Part model, mm, in its own coordinate system. Face numbers are marked on the shaded views. A direction names the side the tool comes from. Round coordinates to 2 decimals unless told otherwise and drop trailing zeros. Write each loop counter-clockwise with the first axis right and the second up, starting at its lowest first coordinate (ties: lowest second). Pieces come first, ordered by that corner, then holes. Notation, with made-up numbers: (55.5, -20) -> (85.5, -20) arc R21 cw to (85.5, -3) -> close; hole circle Ø5 at (26, 61). An arc over 180 degrees is marked (long way). Return JSON: item names as keys, results as strings. Group by question number.
(1) Mould opens along Y. For the marked faces 1, 2 and 3 say: +Y half, -Y half, draft (parallel to the pull), parting line (faces both ways), or undercut.
(2) Tool access for the marked faces 4, 5, 6 and 7: list every direction of +Z, -Z, +X, -X, +Y, -Y with a clear straight run to the whole face (end or side of a thin tool).
(3) Saw through at C-C (x = 165). List the corners of the cut face in (y, z).
(4) Saw through at B-B (x = 75.5). State how many separate pieces and enclosed holes the cut face has, plus the area to 4 significant figures.
(5) Saw through at A-A (z = 12.5). List the corners of the cut face in (x, y).
(6) Drill centre lines: L1, parallel to Y at x = 13.5, z = 29; L2, parallel to Y at x = 13, z = 6.5; L3, parallel to Y at x = 127, z = 57. Where is each one in solid material? Low to high. Write a range as from..to.
(7) Drop flat-ended pins along their axis: pin 1 Ø6 at (x, z) = (-49, 92) entering from +Y; pin 2 Ø4 at (x, y) = (32, 43.5) entering from +Z; pin 3 Ø2 at (x, z) = (168, 18) entering from +Y; pin 4 Ø12 at (x, y) = (17.5, -7) entering from -Z. Give the stop position or say it passes through.
from build123d import *

# Parameters (mm, degrees)
F3_DEPTH = 100
F4_R     = 8.65938
F4_R_2   = 13.370559
F5_DEPTH = 200


with BuildPart() as f1:
    # F0 (on Front) → F1 (revolve)
    with BuildSketch(Plane.XZ):
        Polygon((0, 112.481035), (0, 0), (58.373801, 0), (58.373801, 42.910885), (103.36262, 57.920542), align=None)
    revolve(axis=Axis((0, 0, 56.240518), (0, 0, -1)))

    # F2 (on face) → F3 (cut)
    with BuildSketch(Plane(origin=(0, 0, 0), x_dir=(1, 0, 0), z_dir=(0, 0, -1))):
        with BuildLine():
            Line((0, 28.951159), (0, -28.951159))
            Line((0, -28.951159), (50.68857, -28.951159))
            ThreePointArc((50.68857, -28.951159), (56.419789, -14.976919), (58.373801, 0))
            ThreePointArc((58.373801, 0), (56.419789, 14.976919), (50.68857, 28.951159))
            Line((50.68857, 28.951159), (0, 28.951159))
        make_face()
        with BuildLine():
            ThreePointArc((58.373801, 0), (56.419789, -14.976919), (50.68857, -28.951159))
            Line((50.68857, -28.951159), (267.143011, -28.951159))
            Line((267.143011, -28.951159), (267.143011, 28.951159))
            Line((267.143011, 28.951159), (50.68857, 28.951159))
            ThreePointArc((50.68857, 28.951159), (56.419789, 14.976919), (58.373801, 0))
        make_face()
    extrude(amount=-F3_DEPTH, mode=Mode.SUBTRACT)

    # F4 (on face) → F5 (join)
    with BuildSketch(Plane.YZ):
        with Locations((-9.289023, 57.48608)):
            Circle(F4_R)
        with Locations((-7.069625, 20.480426)):
            Circle(F4_R_2)
    extrude(amount=F5_DEPTH)


solid = f1.part
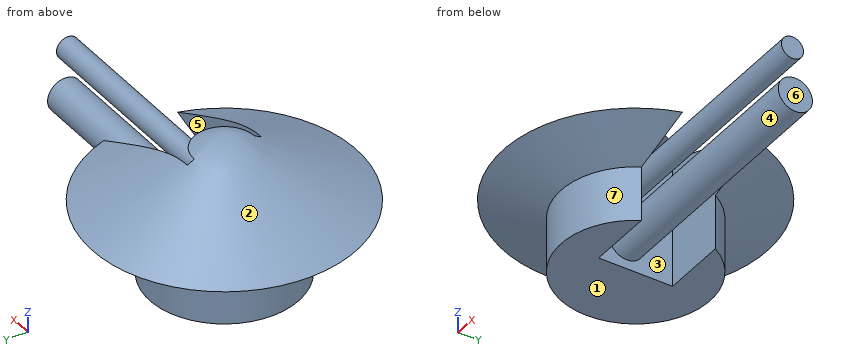
Computed values:
{
 "1": {"face 1": "draft", "face 2": "parting line", "face 3": "undercut"},
 "2": {"face 4": "+X", "face 5": "+Z, -Z, +X", "face 6": "+Z, -Z, +X, +Y, -Y", "face 7": "-Z"},
 "3": {"outline": "circle Ø26.74 at (-7.07, 20.48); circle Ø17.32 at (-9.29, 57.49)"},
 "4": {"separate pieces": "4", "enclosed holes": "0", "area": "1,685 mm2"},
 "5": {"outline": "(0, -28.95) -> (0, -17.8) -> (200, -17.8) -> (200, 3.66) -> (0, 3.66) -> (0, 28.95) -> (50.69, 28.95) arc R58.37 ccw (long way) to (50.69, -28.95) -> close"},
 "6": {"L1": "-56.79..-28.95, -17.37..3.24, 28.95..56.79", "L2": "-56.91..-28.95, 28.95..56.91", "L3": "-17.93..-0.64"},
 "7": {"pin 1": "through", "pin 2": "z = 85.03", "pin 3": "y = 6.22", "pin 4": "z = 7.11"}
}
